Geometry: final body of the model. Coordinates: model frame, mm. A direction names the side the tool comes from. Round coordinates to 2 decimals unless told otherwise and drop trailing zeros. Order: outer loops, then holes, each group sorted by start corner. A loop starts at its lowest first (then second) coordinate and runs counter-clockwise, first axis right, second up. Notation, with made-up numbers: M 32.25,82 L 56.25,82 A17 ccw 56.25,92 Z; hole C 36,89 d10. An arc over 180 degrees is marked long. Put each result on its own line as item: value. Start each with the question number.
1) Section C-C, the plane z = 0.5. Return loops of the section in (x, y).
2) Material intervals for probe 1 along Z at (x, y) = (0.25, 3); probe 2 along Z at (x, y) = (2.5, 4.5); probe 3 along X at (y, z) = (2.25, 3.5), sorted ascending. Write a range as [from, to].
3) Section A-A, the plane y = 2.5. Return loops of the section in (x, z), then the cut area to 3 significant figures.
4) Draft query along X for faces 5 (the flat face through (0, 0, 10)), 6 (the cylindrical face through (2.93, 0.3, 17.85)), 7 (the flat face through (-6, 3, 10)), 8 (the cylindrical face through (2.93, 6.7, 17.85)). Return one class per face: pulls with the +X half, pulls with the -X half, needs draft (parallel to the pull), parting line crosses it, or undercut.
5) Access query for faces 1 (the cylindrical face through (-2.93, 0.3, 2.05)), 2 (the flat face through (0, 3, 4.744)), 3 (the cylindrical face through (0.05, 6.7, 14.97)), 4 (the flat face through (0, 7, 10)). Directions: +Z, -Z, +X, -X, +Y, -Y. A direction counts if a zero-diameter tool reaches every point of the face in a straight line with its end or side. Return the directions, or none.
6) Section B-B, the plane x = 0. Return loops of the section in (y, z).
7) First-contact query: P1, Ø1.5, axis at x = 0.5, y = 5.5, coming from the -Z side. Flat tip, straight axial feed; report the tip coordinate or a pass-through.
8) Section D-D, the plane x = -3.25. Return loops of the section in (y, z), then the cut area to 3 significant figures.
from build123d import *

# Parameters (mm, degrees)
SKETCH4_W           = 5.288
SKETCH4_H           = 5.288
BOSS_EXTRUDE1_DEPTH = 7
FILLET1_R           = 1


with BuildPart() as part:
    # Sketch4 → Boss-Extrude1 (new body)
    with BuildSketch(Plane(origin=(0, 0, 0), x_dir=(1, 0, 0), z_dir=(0, 1, 0))):
        with BuildLine():
            Line((6, 0), (6, -20))
            ThreePointArc((6, -20), (0, -26), (-6, -20))
            Line((-6, -20), (-6, 0))
            ThreePointArc((-6, 0), (0, 6), (6, 0))
        make_face()
        with Locations((0, -17.9)):
            Rectangle(SKETCH4_W, SKETCH4_H, mode=Mode.SUBTRACT)
        with Locations((0, -2.1)):
            Rectangle(SKETCH4_W, SKETCH4_H, mode=Mode.SUBTRACT)
    extrude(amount=BOSS_EXTRUDE1_DEPTH)

    # Fillet1
    fillet1_edges = [part.edges().sort_by_distance(p)[0] for p in [
        (2.644, 0, 2.1),
        (0, 0, -0.544),
        (-2.644, 0, 2.1),
        (0, 0, 4.744),
        (2.644, 7, 2.1),
        (0, 7, -0.544),
        (-2.644, 7, 2.1),
        (0, 7, 4.744),
        (-2.644, 0, 17.9),
        (0, 0, 20.544),
        (2.644, 0, 17.9),
        (0, 0, 15.256),
        (-2.644, 7, 17.9),
        (0, 7, 20.544),
        (2.644, 7, 17.9),
        (0, 7, 15.256),
    ]]
    fillet(fillet1_edges, radius=FILLET1_R)


solid = part.part
Result sheet:
1. outline: M -6,0 L -3.64,0 A1 ccw -2.64,1 L -2.64,6 A1 ccw -3.64,7 L -6,7 Z; M 2.64,1 A1 ccw 3.64,0 L 6,0 L 6,7 L 3.64,7 A1 ccw 2.64,6 Z
2. probe 1: z = [-5.99, -0.54], [4.74, 15.26], [20.54, 25.99]
2. probe 2: z = [-5.45, -0.54], [4.74, 15.26], [20.54, 25.45]
2. probe 3: x = [-6, -2.64], [2.64, 6]
3. outline: M -6,0 A6 ccw 6,0 L 6,20 A6 ccw -6,20 Z; hole M -2.64,-0.54 L 2.64,-0.54 L 2.64,4.74 L -2.64,4.74 Z; hole M -2.64,15.26 L 2.64,15.26 L 2.64,20.54 L -2.64,20.54 Z
3. area: 297 mm2
4. face 5: needs draft
4. face 6: undercut
4. face 7: pulls with the -X half
4. face 8: undercut
5. face 1: -Y
5. face 2: +Y, -Y
5. face 3: +Y
5. face 4: +Z, -Z, +X, -X, +Y
6. outline: M 0,-6 L 7,-6 L 7,-1.54 A1 ccw 6,-0.54 L 1,-0.54 A1 ccw 0,-1.54 Z; M 0,5.74 A1 ccw 1,4.74 L 6,4.74 A1 ccw 7,5.74 L 7,14.26 A1 ccw 6,15.26 L 1,15.26 A1 ccw 0,14.26 Z; M 0,21.54 A1 ccw 1,20.54 L 6,20.54 A1 ccw 7,21.54 L 7,26 L 0,26 Z
7. P1: stops at z = -6
8. outline: M 0,-5.04 L 7,-5.04 L 7,-1.54 A1 ccw 6.92,-1.15 L 6.92,5.35 A1 ccw 7,5.74 L 7,14.26 A1 ccw 6.92,14.65 L 6.92,21.15 A1 ccw 7,21.54 L 7,25.04 L 0,25.04 L 0,21.54 A1 ccw 0.08,21.15 L 0.08,14.65 A1 ccw 0,14.26 L 0,5.74 A1 ccw 0.08,5.35 L 0.08,-1.15 A1 ccw 0,-1.54 Z
8. area: 208 mm2
